The listing builds one solid part. Answer for the finished solid, in the listing's coordinates (mm). A direction names the side the tool comes from. Coordinates: 2 decimals unless noted, no trailing zeros. Order: outer loops, then holes, each group sorted by start corner. A loop starts at its lowest first (then second) coordinate and runs counter-clockwise, first axis right, second up.
Autodesk Inventor part; units mm, degrees
ref_plane "WeldJoint" through (0, 0, -10) normal (0.5299, -0.848, 0) x (0, 0, 1)
ref_plane "Outer" through (0, 0, -10) normal (0.454, -0.891, 0) x (0, 0, 1)
ref_plane "Clock_Feeder" through (0, 0, -10) normal (0, 1, 0) x (0, 0, 1)
sketch "Sketch13" plane through (0, 0, 0) normal (0, 0, 1) x (1, 0, 0)
  circle A0 centre (0, 0) radius 600 construction
  line L0 (0, 0) -> (0, -600)
  line L1 (0, 0) -> (-508.8289, -317.9516)
  line L2 (0, 0) -> (600, 0)
  line L3 (0, 0) -> (0, -600)
  line L4 (0, 0) -> (0, -600)
  line L5 (0, 0) -> (-534.6039, -272.3943)
  arc A1 (-508.8289, -317.9516) -> (0, -600) centre (0, 0) ccw
  dimension "d53" = 1200
  dimension "d54" = 58
  dimension "d55" = 0
  dimension "d56" = 0
  dimension "d57" = 270
  dimension "d58" = 63
ref_plane "WeldJoint" through (0, 0, -10) normal (0.5299, -0.848, 0) x (0, 0, 1)
ref_plane "Outer" through (0, 0, -10) normal (0.454, -0.891, 0) x (0, 0, 1)
ref_plane "Clock_Feeder" through (0, 0, -10) normal (0, 1, 0) x (0, 0, 1)
ref_plane "Charging" through (0, 0, -10) normal (1, 0, 0) x (0, 0, 1)
ref_plane "Accsess" through (0, 0, -10) normal (1, 0, 0) x (0, 0, 1)
sketch "Sketch14" plane through (0, 0, -10) normal (0.5299, -0.848, 0) x (0, 0, 1)
  line L0 (1710, 594) -> (10, 594)
  line L1 (10, 594) -> (10, 600)
  line L2 (10, 600) -> (1710, 600)
  line L3 (1710, 600) -> (1710, 594)
  line L4 (10, 0) -> (825.0673, 0)
  point P0 (10, 597)
  dimension "d59" = 1700
  dimension "d60" = 6
  dimension "d61" = 1200
revolve "Revolution2" add sketch "Sketch14" angle 359.9 about axis through (0, 0, 0) along (0, 0, 1)
sketch "Sketch AnglePlane_Feeder" plane through (0, 0, -10) normal (0, 1, 0) x (0, 0, 1)
  line L0 (10, -600) -> (10, 600)
  line L1 (10, 0) -> (1410, 0)
  line L2 (1410, 0) -> (1410, 600)
  line L3 (1410, 600) -> (10, 600)
  line L4 (10, 600) -> (10, 0)
  point P0 (10, -508.8289)
  point P1 (10, -509.383)
  dimension "d63" = 1200
  dimension "d64" = 90
  dimension "frd_hght" = 1400
ref_plane "AnglePlane_Feeder" through (0, 0, 1400) normal (1, 0, 0) x (0, 1, 0)
sketch "Sketch16" plane through (0, 0, 1400) normal (1, 0, 0) x (0, 1, 0)
  circle A0 centre (0, 0) radius 45.5
  point P0 (0, -1400)
  point P1 (0, 0)
  point P2 (0, 0)
  point P3 (0, 0)
  dimension "d66" = 91
extrude "Extrusion7" cut sketch "Sketch16" along normal through all
ref_plane "Work Plane16" through (0, 0, 0) normal (0, -1, 0) x (1, 0, 0)
sketch "Sketch17" plane through (0, 0, 0) normal (0, -1, 0) x (1, 0, 0)
  circle A0 centre (0, 408.5) radius 268.5
  line L0 (0, 140) -> (-495.5727, 140)
  point P0 (0, 0)
  dimension "d69" = 537
  dimension "d71" = 140
extrude "Extrusion8" cut sketch "Sketch17" along normal through all
sketch "Sketch19" plane through (0, 0, -10) normal (1, 0, 0) x (0, 0, 1)
  line L0 (10, 0) -> (1410, 0)
  line L1 (1410, 0) -> (1410, 600)
  line L2 (1410, 600) -> (10, 600)
  line L3 (10, 600) -> (10, 0)
  dimension "d74" = 1400
  dimension "d76" = 1200
  dimension "d77" = 90
ref_plane "Work Plane18" through (0, 0, 1400) normal (0, -1, 0) x (1, 0, 0)
sketch "Sketch20" plane through (0, 0, 1400) normal (0, -1, 0) x (1, 0, 0)
  line L0 (-103.5, 0) -> (103.5, 0)
  line L1 (103.5, 0) -> (103.5, 125)
  line L2 (103.5, 125) -> (-103.5, 125)
  line L3 (-103.5, 125) -> (-103.5, 0)
  point P0 (0, -1400)
  point P1 (0, 0)
  point P2 (0, 0)
  point P3 (0, 0)
  point P4 (0, 0)
  dimension "d78" = 207
  dimension "d79" = 125
extrude "Extrusion9" cut sketch "Sketch20" along normal through all
equation "\"BendRadius\" = Thickness"
equation "\"BendReliefWidth\" = Thickness"
equation "\"BendReliefDepth\" = 0.5 * Thickness"
equation "\"CornerReliefSize\" = 4 * Thickness"
equation "\"MinimumRemnant\" = 2 * Thickness"
equation "\"TransitionRadius\" = BendRadius"
equation "\"JacobiRadiusSize\" = BendRadius"
equation "\"GapSize\" = Thickness"
equation "\"Feeder_horisont_angle\" = 0"
equation "\"Hatch_Accsess_diameter\" = 535"
equation "\"Clock_Accsess_angle\" = 0"
equation "\"Clock_Charging_agnle\" = 0"
equation "\"Clock_Feeder_angle\" = 270deg"
equation "\"Clock_Outer_angle\" = 63deg"
equation "\"Clock_WeldJoint_angle\" = 58deg"
properties part number "PRS 1200-10 main Shell" material "Steel"
(1) Find section D-D (x = 0). Write down the section's boundary in (y, z).
(2) Find section B-B (x = 365). Write down the section's boundary in (y, z), and give its area (3 significant figures).
(3) Find section A-A (y = 0). Write down the section's boundary in (x, z), and give its area (3 significant figures).
(4) Each of these flat-tipped pins is pushed along its axis until it touches: pin 1 Ø3 at (y, z) = (72.5, 1104) entering from -X; pin 2 Ø10 at (x, z) = (69, 1237) entering from +Y; pin 3 Ø2 at (y, z) = (-401.5, 1334) entering from +X. Where does it stop, or does it pass through?
(5) For faces 1 (the face through (181.373, -567.36, 606.48)), 2 (the face through (423, -420, 1700)), determine the directions among +Z, -Z, +X, -X, +Y, -Y from which every point of the face is accessible in a straight line to the end or side of a thin tool.
(6) The mould has two halves that part along Y. Classify faces 3 (the face through (596.073, -36.107, 1427.686)), 4 (the face through (210.91, 561.71, 861.9)), 5 (the face through (423, -420, 0)): released by +Y, released by -Y, zero draft, split by the parting line, or undercut.
(7) Find section C-C (z = 408.5). Write down the section's boundary in (x, y).
(8) Consider line 1 (X direction, y = 20.5, z = 494); line 2 (X direction, y = -14.5, z = 1202.5); line 3 (Y direction, x = 412.5, z = 1451). Determine where each line is inside the solid, lowest interval first.
Findings below:
1. outline: (-600, 0) - (-594, 0) - (-594, 140) - (-600, 140) - close; (-600, 677) - (-594, 677) - (-594, 1400) - (-600, 1400) - close; (-600, 1525) - (-594, 1525) - (-594, 1700) - (-600, 1700) - close; (594, 0) - (600, 0) - (600, 1700) - (594, 1700) - close
2. outline: (-476.21, 0) - (-468.63, 0) - (-468.63, 1700) - (-476.21, 1700) - close; (468.63, 0) - (476.21, 0) - (476.21, 1700) - (468.63, 1700) - close
2. area: 25,800 mm2
3. outline: (-600, 0) - (-594, 0) - (-594, 1700) - (-600, 1700) - close; (594, 0) - (600, 0) - (600, 1354.5) - (594, 1354.5) - close; (594, 1445.5) - (600, 1445.5) - (600, 1700) - (594, 1700) - close
3. area: 19,900 mm2
4. pin 1: stops at x = -595.78
4. pin 2: stops at y = 596.58
4. pin 3: stops at x = 446.77
5. face 1: -Y
5. face 2: +Z, +X, -X, +Y, -Y
6. face 3: undercut
6. face 4: split by the parting line
6. face 5: zero draft
7. outline: (-509.38, -317.06) - (-504.29, -313.89) arc R594 cw (long way) to (268.5, -529.85) - (268.5, -536.57) arc R600 ccw (long way) to start; (-508.83, -317.95) arc R600 ccw to (-268.5, -536.57) - (-268.5, -529.85) arc R594 cw to (-503.74, -314.77) - close
8. line 1: x = -599.65 to -593.65, 593.65 to 599.65
8. line 2: x = -599.82 to -593.82, 593.82 to 599.82
8. line 3: y = -435.71 to -427.41, 427.41 to 435.71
